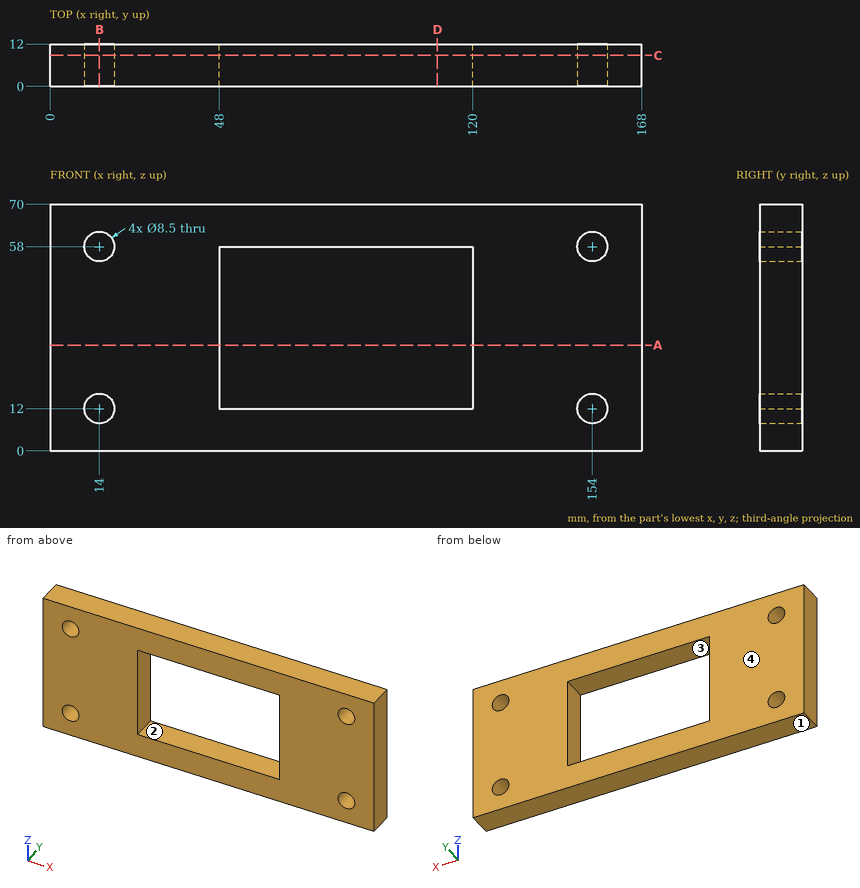
Print and shaded views of the part. All mm, measured from the part's lowest x, y and z. A direction names the side the tool comes from. Coordinates: 2 decimals unless noted, no trailing zeros. Write each loop counter-clockwise with the first axis right and the second up, starting at its lowest first coordinate (ties: lowest second). Pieces come first, ordered by that corner, then holes.
(1) 3-axis set-ups, long thin cutter, end or side, ignore diameter. For the marked faces 1 and 2: which of +Z, -Z, +X, -X, +Y, -Y reach the whole face in a straight line?
(2) Cut at D-D, the plane x = 110. List the corners of the cut face in (y, z).
(3) Cut at A-A, the plane z = 30. List the corners of the cut face in (x, y).
(4) Flat gauge pin, fed straight in: pin 1 (7.5 mm diameter, centred on x = 154, z = 12, fed in from -Y). Where does the tip first touch, or does it go through?
(5) Cut at B-B, the plane x = 14. List the corners of the cut face in (y, z).
(6) Cut at C-C, the plane y = 8.75. List the corners of the cut face in (x, z).
(7) Two-plate mould, pull along X, no slides. Class the marked faces 3 and 4: +X half, -X half, draft (parallel to the pull), parting line (faces both ways), or undercut.
(8) Drill centre lines: probe 1 along X at (y, z) = (6.25, 48); probe 2 along X at (y, z) = (10.5, 9); probe 3 along Z at (x, y) = (79.5, 2.5). Where is each one in solid material? Low to high.
Geometry says:
1. face 1: -Z, +X, -X, +Y, -Y
1. face 2: +Y, -Y
2. outline: (0, 0) - (12, 0) - (12, 12) - (0, 12) - close; (0, 58) - (12, 58) - (12, 70) - (0, 70) - close
3. outline: (0, 0) - (48, 0) - (48, 12) - (0, 12) - close; (120, 0) - (168, 0) - (168, 12) - (120, 12) - close
4. pin 1: passes through
5. outline: (0, 0) - (12, 0) - (12, 7.75) - (0, 7.75) - close; (0, 16.25) - (12, 16.25) - (12, 53.75) - (0, 53.75) - close; (0, 62.25) - (12, 62.25) - (12, 70) - (0, 70) - close
6. outline: (0, 0) - (168, 0) - (168, 70) - (0, 70) - close; hole circle Ø8.5 at (14, 12); hole circle Ø8.5 at (14, 58); hole (48, 12) - (120, 12) - (120, 58) - (48, 58) - close; hole circle Ø8.5 at (154, 12); hole circle Ø8.5 at (154, 58)
7. face 3: undercut
7. face 4: draft
8. probe 1: x = 0 to 48, 120 to 168
8. probe 2: x = 0 to 10.99, 17.01 to 150.99, 157.01 to 168
8. probe 3: z = 0 to 12, 58 to 70
